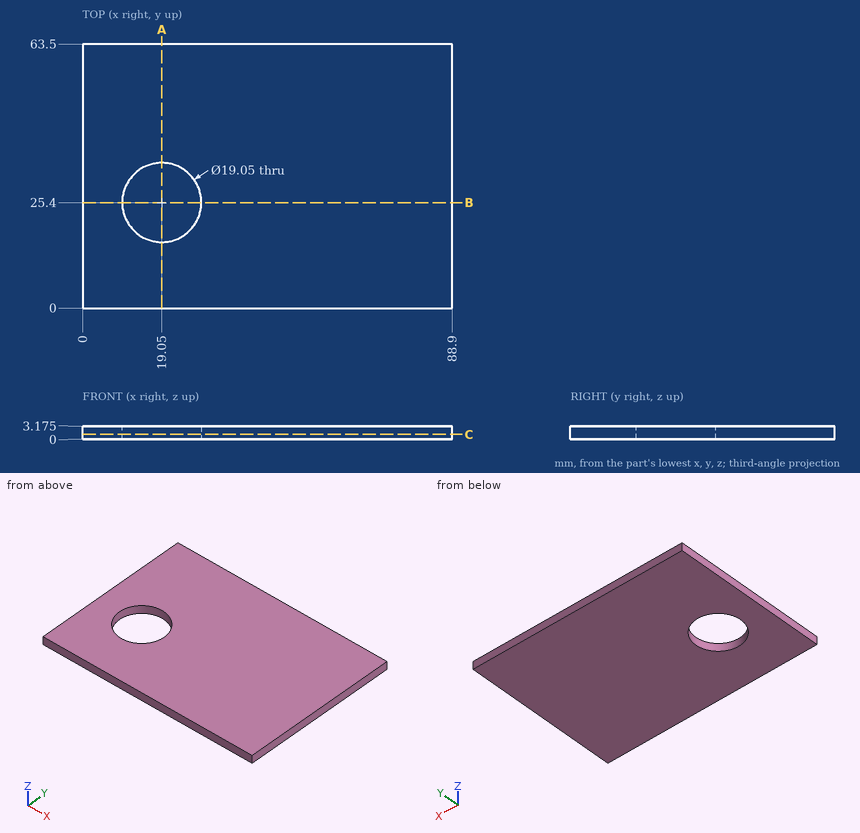
Part print with two shaded views. Sizes in mm from the minimum x, y, z corner. Give positions to 0.01 mm unless a question says otherwise; leave off trailing zeros. Order: outer loops, then holes, each group sorted by start corner. A loop starts at its lowest first (then second) coordinate and runs counter-clockwise, first axis right, second up. Notation, with made-up numbers: M 24.25,-32.5 L 36.25,-32.5 A30 ccw 36.25,-3.5 Z; hole C 89.25,25 d4. An arc over 180 degrees is marked long. Put each result on its own line as item: value.
Item 1: Cut at A-A on x = 19.05. Write the cut outline in (y, z) (3 decimals), then the cut area to 3 significant figures.
Results are:
outline: M 0,0 L 15.875,0 L 15.875,3.175 L 0,3.175 Z; M 34.925,0 L 63.5,0 L 63.5,3.175 L 34.925,3.175 Z
area: 141 mm2
Item 2: Cut at C-C on z = 1.2. Write the cut outline in (x, y) (3 decimals), then the cut area to 3 significant figures.
Results are:
outline: M 0,0 L 88.9,0 L 88.9,63.5 L 0,63.5 Z; hole C 19.05,25.4 d19.05
area: 5,360 mm2
Item 3: Cut at B-B on y = 25.4. Write the cut outline in (x, z) (3 decimals).
Results are:
outline: M 0,0 L 9.525,0 L 9.525,3.175 L 0,3.175 Z; M 28.575,0 L 88.9,0 L 88.9,3.175 L 28.575,3.175 Z
Item 4: Wall check: probe 1 along Y at (x, z) = (19.05, 1.3) (3 decimals); probe 2 along Y at (x, z) = (27, 2.5); probe 3 along X at (y, z) = (34, 0.2). Give the ranges that are in metal, low to high.
Results are:
probe 1: 0 to 15.875, 34.925 to 63.5
probe 2: 0 to 20.15, 30.65 to 63.5
probe 3: 0 to 14.96, 23.14 to 88.9
